Source: CAD feature listing. Evaluate the final solid. Frame: model axes, mm. Face numbers are marked on the shaded views. A direction names the side the tool comes from. Give positions to 0.01 mm unless a question says otherwise; leave off trailing zeros. Order: outer loops, then holes, each group sorted by start corner. A loop starts at its lowest first (then second) coordinate and runs counter-clockwise, first axis right, second up. Notation, with made-up numbers: (-14, 86.5) - (42, 86.5) arc R8 cw to (42, 91.5) - close; hole circle Ø5 at (72.5, 59). An arc over 180 degrees is marked (long way). Use CSV: the item, a comma, the result in double quotes.
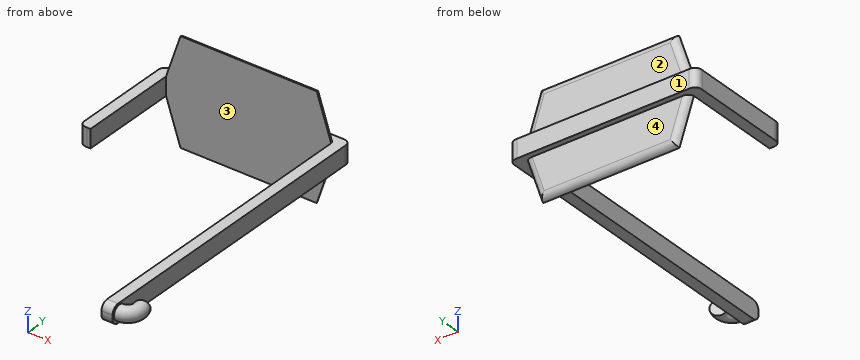
```python
from build123d import *

# Parameters (mm, degrees)
F0_W         = 3
F0_H         = 27
F1_DEPTH     = 5
F3_DEPTH     = 1.5
F4_R         = 2
F5_ANGLE     = 116.8724050768
F6_R         = 2
F7_T1_DEPTH  = 15
F7_T3_DEPTH  = 46.8093211895
F7_T8_DEPTH  = 22.1126839652
F7_T13_DEPTH = 22.1126839652
F7_T18_DEPTH = 22.1126839652
F7_T23_DEPTH = 22.1126839652
F7_T28_DEPTH = 22.1126839652
F7_T33_DEPTH = 22.1126839652
F7_T38_DEPTH = 22.1126839652
F7_T43_DEPTH = 22.1126839652


# Not quite as in the source:
# - a fillet or chamfer that OpenCascade refuses, or shapes differently, is made with other operations: its cross-section is extruded or revolved along the edge and cut away or added


with BuildPart() as f1:
    # F0 (on Top) → F1 (new body)
    with BuildSketch(Plane.XY):
        Polygon((1.5, -42.5), (1.5, 42.5), (-1.5, 42.5), (-1.5, 39.5), (-1.5, -42.5), align=None)
        Polygon((-1.5, 39.5), (-1.5, 42.5), (-49.5, 42.5), (-49.5, 39.5), (-46.5, 39.5), align=None)
        with Locations((-48, 26)):
            Rectangle(F0_W, F0_H)
    extrude(amount=F1_DEPTH)

    # F2 (on face) → F3 (join)
    with BuildSketch(Plane.XZ.offset(-39.5)):
        Polygon((-42.563431412, 16.7904171348), (-46.5, 5), (-1.5, 5), (-5.436568588, 16.7904171348), (-24, 16.7904171348), align=None)
        Polygon((-1.5, 0), (-46.5, 0), (-42.563431412, -11.7904171348), (-24, -11.7904171348), (-5.436568588, -11.7904171348), align=None)
    extrude(amount=-F3_DEPTH)

    # F4 (on face) → F5 (revolve)
    with BuildSketch(Plane.YZ.offset(1.5)):
        with Locations((-40, 2.5)):
            Circle(F4_R)
    revolve(axis=Axis((1.5, -37, 2.371235867), (0, 0, 1)), revolution_arc=F5_ANGLE)

    # F6
    f6_edges = [f1.edges().sort_by_distance(p)[0] for p in [
        (0, -42.5, 0),
        (0, -42.5, 5),
    ]]
    fillet(f6_edges, radius=F6_R)

    # F7: fillet of radius 2 on 9 edges, made by hand

    # F7_s2 → F7_t1 (cut)
    with BuildSketch(Plane.XY.offset(-5)):
        with BuildLine():
            add(Edge.make_bspline(
                [(1.5, 40.5), (1.5, 42.5), (-0.5, 42.5)],
                knots=[0, 0, 0, 1, 1, 1], degree=2, weights=[1, 1, 1]))
            Line((-0.5, 42.5), (1.5, 42.5))
            Line((1.5, 42.5), (1.5, 40.5))
        make_face()
        with BuildLine():
            add(Edge.make_bspline(
                [(-47.5, 42.5), (-49.5, 42.5), (-49.5, 40.5)],
                knots=[0, 0, 0, 1, 1, 1], degree=2, weights=[1, 1, 1]))
            Line((-49.5, 40.5), (-49.5, 42.5))
            Line((-49.5, 42.5), (-47.5, 42.5))
        make_face()
        with BuildLine():
            add(Edge.make_bspline(
                [(-49.5, 14.5), (-49.5, 12.5), (-47.5, 12.5)],
                knots=[0, 0, 0, 1, 1, 1], degree=2, weights=[1, 1, 1]))
            Line((-47.5, 12.5), (-49.5, 12.5))
            Line((-49.5, 12.5), (-49.5, 14.5))
        make_face()
    extrude(amount=F7_T1_DEPTH, mode=Mode.SUBTRACT)

    # F7_s4 → F7_t3 (cut)
    with BuildSketch(Plane.YZ.offset(-47.4046605947)):
        with BuildLine():
            add(Edge.make_bspline(
                [(41, 14.8539254617), (41, 16.4031188001), (39.5, 16.7904171348)],
                knots=[0, 0, 0, 1, 1, 1], degree=2, weights=[1, 1, 1]))
            Line((39.5, 16.7904171348), (41, 16.7904171348))
            Line((41, 16.7904171348), (41, 14.8539254617))
        make_face()
        with BuildLine():
            add(Edge.make_bspline(
                [(41, -9.8539254617), (41, -11.4031188001), (39.5, -11.7904171348)],
                knots=[0, 0, 0, 1, 1, 1], degree=2, weights=[1, 1, 1]))
            Line((39.5, -11.7904171348), (41, -11.7904171348))
            Line((41, -11.7904171348), (41, -9.8539254617))
        make_face()
    extrude(amount=F7_T3_DEPTH, mode=Mode.SUBTRACT)


with BuildPart() as f7_tool6:
    # F7_s7 → F7_t8 (new body)
    with BuildSketch(Plane(origin=(2.3080156307, 0, 6.912737942), x_dir=(0, 1, 0), z_dir=(-0.3166932536, 0, -0.9485280086))):
        with BuildLine():
            add(Edge.make_bspline(
                [(41, -43.7535269955), (41, -45.302720334), (39.5, -45.6900186686)],
                knots=[0, 0, 0, 1, 1, 1], degree=2, weights=[1, 1, 1]))
            Line((39.5, -45.6900186686), (41, -45.6900186686))
            Line((41, -45.6900186686), (41, -43.7535269955))
        make_face()
    extrude(amount=F7_T8_DEPTH)

    split(bisect_by=Plane.XY.offset(5), keep=Keep.TOP)


with BuildPart() as f1_1:
    add(f1.part)

    # F7_t5: cut F7_tool6
    add(f7_tool6.part, mode=Mode.SUBTRACT)


with BuildPart() as f7_tool11:
    # F7_s12 → F7_t13 (new body)
    with BuildSketch(Plane(origin=(2.3080156307, 0, 6.912737942), x_dir=(0, 1, 0), z_dir=(-0.3166932536, 0, -0.9485280086))):
        with BuildLine():
            add(Edge.make_bspline(
                [(41, -43.7535269955), (41, -45.302720334), (39.5, -45.6900186686)],
                knots=[0, 0, 0, 1, 1, 1], degree=2, weights=[1, 1, 1]))
            Line((39.5, -45.6900186686), (41, -45.6900186686))
            Line((41, -45.6900186686), (41, -43.7535269955))
        make_face()
    extrude(amount=F7_T13_DEPTH)

    split(bisect_by=Plane.XY, keep=Keep.BOTTOM)


with BuildPart() as f1_2:
    add(f1_1.part)

    # F7_t10: cut F7_tool11
    add(f7_tool11.part, mode=Mode.SUBTRACT)


with BuildPart() as f7_tool16:
    # F7_s17 → F7_t18 (new body)
    with BuildSketch(Plane(origin=(-0.1192194099, 0, 0.3570740714), x_dir=(0, 1, 0), z_dir=(-0.3166932536, 0, 0.9485280086))):
        with BuildLine():
            add(Edge.make_bspline(
                [(39.5, -0.160674255), (41, 0.2266240796), (41, 1.7758174181)],
                knots=[0, 0, 0, 1, 1, 1], degree=2, weights=[1, 1, 1]))
            Line((41, 1.7758174181), (41, -0.160674255))
            Line((41, -0.160674255), (39.5, -0.160674255))
        make_face()
    extrude(amount=F7_T18_DEPTH)

    split(bisect_by=Plane.XY, keep=Keep.BOTTOM)


with BuildPart() as f1_3:
    add(f1_2.part)

    # F7_t15: cut F7_tool16
    add(f7_tool16.part, mode=Mode.SUBTRACT)


with BuildPart() as f7_tool21:
    # F7_s22 → F7_t23 (new body)
    with BuildSketch(Plane(origin=(-0.1192194099, 0, 0.3570740714), x_dir=(0, 1, 0), z_dir=(-0.3166932536, 0, 0.9485280086))):
        with BuildLine():
            add(Edge.make_bspline(
                [(39.5, -0.160674255), (41, 0.2266240796), (41, 1.7758174181)],
                knots=[0, 0, 0, 1, 1, 1], degree=2, weights=[1, 1, 1]))
            Line((41, 1.7758174181), (41, -0.160674255))
            Line((41, -0.160674255), (39.5, -0.160674255))
        make_face()
    extrude(amount=F7_T23_DEPTH)

    split(bisect_by=Plane.XY.offset(5), keep=Keep.TOP)


with BuildPart() as f1_4:
    add(f1_3.part)

    # F7_t20: cut F7_tool21
    add(f7_tool21.part, mode=Mode.SUBTRACT)


with BuildPart() as f7_tool26:
    # F7_s27 → F7_t28 (new body)
    with BuildSketch(Plane(origin=(-6.1968843057, 0, 18.5602890603), x_dir=(0, 1, 0), z_dir=(0.3166932536, 0, -0.9485280086))):
        with BuildLine():
            add(Edge.make_bspline(
                [(41, -42.1700607276), (41, -43.7192540661), (39.5, -44.1065524007)],
                knots=[0, 0, 0, 1, 1, 1], degree=2, weights=[1, 1, 1]))
            Line((39.5, -44.1065524007), (41, -44.1065524007))
            Line((41, -44.1065524007), (41, -42.1700607276))
        make_face()
    extrude(amount=F7_T28_DEPTH)

    split(bisect_by=Plane.XY.offset(5), keep=Keep.TOP)


with BuildPart() as f1_5:
    add(f1_4.part)

    # F7_t25: cut F7_tool26
    add(f7_tool26.part, mode=Mode.SUBTRACT)


with BuildPart() as f7_tool31:
    # F7_s32 → F7_t33 (new body)
    with BuildSketch(Plane(origin=(-6.1968843057, 0, 18.5602890603), x_dir=(0, 1, 0), z_dir=(0.3166932536, 0, -0.9485280086))):
        with BuildLine():
            add(Edge.make_bspline(
                [(41, -42.1700607276), (41, -43.7192540661), (39.5, -44.1065524007)],
                knots=[0, 0, 0, 1, 1, 1], degree=2, weights=[1, 1, 1]))
            Line((39.5, -44.1065524007), (41, -44.1065524007))
            Line((41, -44.1065524007), (41, -42.1700607276))
        make_face()
    extrude(amount=F7_T33_DEPTH)

    split(bisect_by=Plane.XY, keep=Keep.BOTTOM)


with BuildPart() as f1_6:
    add(f1_5.part)

    # F7_t30: cut F7_tool31
    add(f7_tool31.part, mode=Mode.SUBTRACT)


with BuildPart() as f7_tool36:
    # F7_s37 → F7_t38 (new body)
    with BuildSketch(Plane(origin=(-5.6201951346, 0, -16.8330472425), x_dir=(0, 1, 0), z_dir=(0.3166932536, 0, 0.9485280086))):
        with BuildLine():
            add(Edge.make_bspline(
                [(39.5, 1.4227920129), (41, 1.8100903475), (41, 3.359283686)],
                knots=[0, 0, 0, 1, 1, 1], degree=2, weights=[1, 1, 1]))
            Line((41, 3.359283686), (41, 1.4227920129))
            Line((41, 1.4227920129), (39.5, 1.4227920129))
        make_face()
    extrude(amount=F7_T38_DEPTH)

    split(bisect_by=Plane.XY, keep=Keep.BOTTOM)


with BuildPart() as f1_7:
    add(f1_6.part)

    # F7_t35: cut F7_tool36
    add(f7_tool36.part, mode=Mode.SUBTRACT)


with BuildPart() as f7_tool41:
    # F7_s42 → F7_t43 (new body)
    with BuildSketch(Plane(origin=(-5.6201951346, 0, -16.8330472425), x_dir=(0, 1, 0), z_dir=(0.3166932536, 0, 0.9485280086))):
        with BuildLine():
            add(Edge.make_bspline(
                [(39.5, 1.4227920129), (41, 1.8100903475), (41, 3.359283686)],
                knots=[0, 0, 0, 1, 1, 1], degree=2, weights=[1, 1, 1]))
            Line((41, 3.359283686), (41, 1.4227920129))
            Line((41, 1.4227920129), (39.5, 1.4227920129))
        make_face()
    extrude(amount=F7_T43_DEPTH)

    split(bisect_by=Plane.XY.offset(5), keep=Keep.TOP)


with BuildPart() as f1_8:
    add(f1_7.part)

    # F7_t40: cut F7_tool41
    add(f7_tool41.part, mode=Mode.SUBTRACT)


solid = f1_8.part
```
Item 1: First-contact query: pin 1 (1.5 mm diameter, centred on x = -3.5, y = -13, fed in from -Z); pin 2 (12 mm diameter, centred on y = 29.5, z = 5.5, fed in from +X); pin 3 (8 mm diameter, centred on x = -18.5, z = -7.5, fed in from +Y); pin 4 (12 mm diameter, centred on x = -33, z = -7.5, fed in from -Y). Flat tips, straight axial feed; report the tip coordinate or a pass-through.
Filled in:
pin 1,"passes through"
pin 2,"stops at x = 1.5"
pin 3,"stops at y = 41"
pin 4,"stops at y = 39.5"
Item 2: Section A-A on y = 18. Return the cut outline in (x, z).
Filled in:
outline,"(-49.5, 0) - (-46.5, 0) - (-46.5, 5) - (-49.5, 5) - close; (-1.5, 0) - (1.5, 0) - (1.5, 5) - (-1.5, 5) - close"
Item 3: Material intervals for line 1 (Y direction, x = -37, z = 8.25); line 2 (X direction, y = 20, z = 1); line 3 (Z direction, x = 0, y = 27.5), sorted ascending. Write a range as from..to.
Filled in:
line 1,"y = 39.5..41"
line 2,"x = -49.5..-46.5, -1.5..1.5"
line 3,"z = 0..5"
Item 4: Mould query, pull axis X, two halves, no side actions, for the marked faces 3 and 4. Classes: released by +X, released by -X, zero draft, split by the parting line, or undercut.
Filled in:
face 3,"undercut"
face 4,"zero draft"
Item 5: Set-up query: the marked faces 1 and 2. Return all of +Z, -Z, +X, -X, +Y, -Y with unobstructed straight access to the full face (end or side cutting, diameter ignored); none if empty.
Filled in:
face 1,"+Z, -Z, +X, -X, +Y"
face 2,"+Z, +X, -X, +Y"
Item 6: Section B-B on y = -15. Return the cut outline in (x, z).
Filled in:
outline,"(-1.5, 0) - (1.5, 0) - (1.5, 5) - (-1.5, 5) - close"
